Answer from the drawing. Dimensions are ordinates in mm from the lowest x, y and z of the part. A direction names the side the tool comes from. Coordinates: 2 decimals unless noted, no trailing zeros. Loops run counter-clockwise (first coordinate to the right, second up) from the corner with the lowest first, then second, coordinate; pieces in that order, holes last. Notation, with made-up numbers: (-5, -17) - (53, -17) arc R19 ccw to (53, 2) - close; hole circle Ø8 at (46, -28). An arc over 180 degrees is marked (long way). Write each question's results on one line, items separated by ' | '. Start each with the question number.
1. A cutting plane is placed at B-B on x = 153. Determine the outline of the cut face in (y, z).
2. Find the intervals of material crossed by line 1 along Y through (x, z) = (71, 10); line 2 along X through (y, z) = (72.5, 5.25); line 3 along Y through (x, z) = (27, 4), in increasing order. Write a range as [from, to].
3. A cutting plane is placed at C-C on y = 88. State how many separate pieces and enclosed holes the cut face has, then the cut area to 3 significant figures.
4. Which of the six approach directions +Z, -Z, +X, -X, +Y, -Y give full straight-line access (tool end or side, diameter ignored) to the marked faces 4, 5 and 6?
5. Determine the mould class of the marked faces 1, 2 and 3 for opening direction Y: released by +Y, released by -Y, zero draft, split by the parting line, or undercut.
6. This flat-tipped pin is pushed along its axis until it touches: P1, Ø0.6, axis at x = 112, z = 17.5, coming from the -Y side. Where does it stop, or does it pass through?
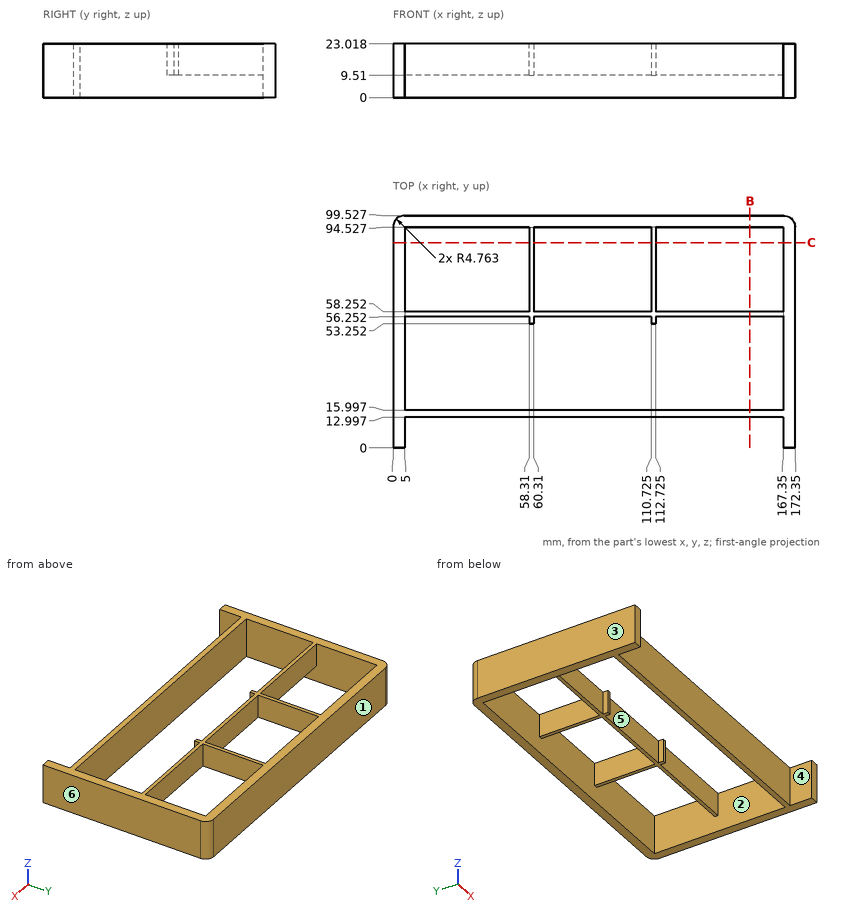
Values:
1) outline: (13, 0) - (16, 0) - (16, 23.02) - (13, 23.02) - close; (56.25, 9.51) - (58.25, 9.51) - (58.25, 23.02) - (56.25, 23.02) - close; (94.53, 0) - (99.53, 0) - (99.53, 23.02) - (94.53, 23.02) - close
2) line 1: [13, 16], [56.25, 58.25], [94.53, 99.53] | line 2: [0, 5], [167.35, 172.35] | line 3: [13, 16], [94.53, 99.53]
3) separate pieces: 4 | enclosed holes: 0 | area: 284 mm^2
4) face 4: +Z, -Z, -Y | face 5: +Z, -Z | face 6: +Z, -Z, +X, +Y, -Y
5) face 1: released by +Y | face 2: undercut | face 3: zero draft
6) P1: y = 13
